The model under review builds one solid part; all positions refer to its coordinate system, in mm. Face numbers are marked on the shaded views. Round coordinates to 2 decimals unless told otherwise and drop trailing zeros. Loops run counter-clockwise (first coordinate to the right, second up) from the corner with the lowest first, then second, coordinate; pieces in that order, holes last. Notation, with made-up numbers: (-32.5, -18.75) -> (-6.5, -18.75) arc R14 ccw to (-6.5, -4.75) -> close; hole circle Ø7 at (3.5, 51). An arc over 180 degrees is marked (long way). Return JSON: item names as keys, results as strings. Group by question number.
```python
from build123d import *

# Parameters (mm, degrees)
F0_R     = 4.493782
F0_R_2   = 8.414158
F0_R_3   = 6.15385
F0_R_4   = 6.841255
F1_DEPTH = 6.35


with BuildPart() as f1:
    # F0 (on Front) → F1 (new body, symmetric)
    with BuildSketch(Plane.XZ):
        with BuildLine():
            Line((0, 9.352685), (0, 69.849999))
            ThreePointArc((0, 69.849999), (-26.730437, 64.532984), (-49.391408, 49.391408))
            Line((-49.391408, 49.391408), (-6.613347, 6.613347))
            ThreePointArc((-6.613347, 6.613347), (-3.579118, 8.640754), (0, 9.352685))
        make_face()
        with Locations((-9.287155, 20.851616)):
            Circle(F0_R, mode=Mode.SUBTRACT)
        with Locations((-19.314256, 38.508028)):
            Circle(F0_R_2, mode=Mode.SUBTRACT)
        with Locations((-36.098748, 50.714932)):
            Circle(F0_R_3, mode=Mode.SUBTRACT)
        with Locations((-12.992823, 59.434153)):
            Circle(F0_R_4, mode=Mode.SUBTRACT)
        with BuildLine():
            Line((7.121327, 6.062955), (49.917759, 48.859387))
            ThreePointArc((49.917759, 48.859387), (27.075766, 64.388859), (0, 69.849999))
            Line((0, 69.849999), (0, 9.352685))
            ThreePointArc((0, 9.352685), (3.922232, 8.490513), (7.121327, 6.062955))
        make_face()
        with Locations((9.287155, 20.851616)):
            Circle(F0_R, mode=Mode.SUBTRACT)
        with Locations((19.314256, 38.508028)):
            Circle(F0_R_2, mode=Mode.SUBTRACT)
        with Locations((36.098748, 50.714932)):
            Circle(F0_R_3, mode=Mode.SUBTRACT)
        with Locations((12.992823, 59.434153)):
            Circle(F0_R_4, mode=Mode.SUBTRACT)
        with BuildLine():
            Line((48.668913, 0), (69.849999, 0))
            ThreePointArc((69.849999, 0), (64.675257, 26.384341), (49.917759, 48.859387))
            Line((49.917759, 48.859387), (7.121327, 6.062955))
            ThreePointArc((7.121327, 6.062955), (8.777136, 3.230262), (9.352685, 0))
            Line((9.352685, 0), (33.899703, 0))
            ThreePointArc((33.899703, 0), (41.284308, 7.384605), (48.668913, 0))
        make_face()
        with Locations((21.909988, 8.228783)):
            Circle(F0_R, mode=Mode.SUBTRACT)
        with Locations((39.5664, 18.255884)):
            Circle(F0_R_2, mode=Mode.SUBTRACT)
        with Locations((60.492525, 11.934451)):
            Circle(F0_R_4, mode=Mode.SUBTRACT)
        with Locations((51.773304, 35.040376)):
            Circle(F0_R_3, mode=Mode.SUBTRACT)
        with BuildLine():
            ThreePointArc((57.120882, -40.202329), (66.591726, -21.084696), (69.849999, 0))
            Line((69.849999, 0), (48.668913, 0))
            ThreePointArc((48.668913, 0), (41.284308, -7.384605), (33.899703, 0))
            Line((33.899703, 0), (9.352685, 0))
            ThreePointArc((9.352685, 0), (8.640754, -3.579118), (6.613347, -6.613347))
            Line((6.613347, -6.613347), (49.391408, -49.391408))
            ThreePointArc((49.391408, -49.391408), (53.037147, -45.45419), (56.369892, -41.248728))
            ThreePointArc((56.369892, -41.248728), (46.021931, -34.968153), (57.927155, -37.15712))
            ThreePointArc((57.927155, -37.15712), (57.722172, -38.732189), (57.120882, -40.202329))
        make_face()
        with Locations((21.909988, -10.345527)):
            Circle(F0_R, mode=Mode.SUBTRACT)
        with Locations((39.5664, -20.372628)):
            Circle(F0_R_2, mode=Mode.SUBTRACT)
        with Locations((60.492525, -14.051196)):
            Circle(F0_R_4, mode=Mode.SUBTRACT)
        with BuildLine():
            ThreePointArc((41.248728, -56.369892), (45.45419, -53.037147), (49.391408, -49.391408))
            Line((49.391408, -49.391408), (6.613347, -6.613347))
            ThreePointArc((6.613347, -6.613347), (3.579118, -8.640754), (0, -9.352685))
            Line((0, -9.352685), (0, -69.849999))
            ThreePointArc((0, -69.849999), (21.084696, -66.591726), (40.202329, -57.120882))
            ThreePointArc((40.202329, -57.120882), (31.836894, -48.680561), (43.310971, -51.773304))
            ThreePointArc((43.310971, -51.773304), (42.771789, -54.292305), (41.248728, -56.369892))
        make_face()
        with Locations((14.051196, -60.492525)):
            Circle(F0_R_4, mode=Mode.SUBTRACT)
        with Locations((20.372628, -39.5664)):
            Circle(F0_R_2, mode=Mode.SUBTRACT)
        with Locations((10.345527, -21.909988)):
            Circle(F0_R, mode=Mode.SUBTRACT)
        with BuildLine():
            ThreePointArc((-48.859387, -49.917759), (-26.384341, -64.675257), (0, -69.849999))
            Line((0, -69.849999), (0, -9.352685))
            ThreePointArc((0, -9.352685), (-3.230262, -8.777136), (-6.062955, -7.121327))
            Line((-6.062955, -7.121327), (-48.859387, -49.917759))
        make_face()
        with Locations((-11.934451, -60.492525)):
            Circle(F0_R_4, mode=Mode.SUBTRACT)
        with Locations((-35.040376, -51.773304)):
            Circle(F0_R_3, mode=Mode.SUBTRACT)
        with Locations((-18.255884, -39.5664)):
            Circle(F0_R_2, mode=Mode.SUBTRACT)
        with Locations((-8.228783, -21.909988)):
            Circle(F0_R, mode=Mode.SUBTRACT)
        with BuildLine():
            ThreePointArc((-69.849999, 0), (-64.388859, -27.075766), (-48.859387, -49.917759))
            Line((-48.859387, -49.917759), (-6.062955, -7.121327))
            ThreePointArc((-6.062955, -7.121327), (-8.490513, -3.922232), (-9.352685, 0))
            Line((-9.352685, 0), (-33.899703, 0))
            ThreePointArc((-33.899703, 0), (-41.284308, -7.384605), (-48.668913, 0))
            Line((-48.668913, 0), (-69.849999, 0))
        make_face()
        with Locations((-50.714932, -36.098748)):
            Circle(F0_R_3, mode=Mode.SUBTRACT)
        with Locations((-38.508028, -19.314256)):
            Circle(F0_R_2, mode=Mode.SUBTRACT)
        with Locations((-59.434153, -12.992823)):
            Circle(F0_R_4, mode=Mode.SUBTRACT)
        with Locations((-20.851616, -9.287155)):
            Circle(F0_R, mode=Mode.SUBTRACT)
        with BuildLine():
            Line((-6.613347, 6.613347), (-49.391408, 49.391408))
            ThreePointArc((-49.391408, 49.391408), (-64.532984, 26.730437), (-69.849999, 0))
            Line((-69.849999, 0), (-48.668913, 0))
            ThreePointArc((-48.668913, 0), (-41.284308, 7.384605), (-33.899703, 0))
            Line((-33.899703, 0), (-9.352685, 0))
            ThreePointArc((-9.352685, 0), (-8.640754, 3.579118), (-6.613347, 6.613347))
        make_face()
        with Locations((-59.434153, 12.992823)):
            Circle(F0_R_4, mode=Mode.SUBTRACT)
        with Locations((-38.508028, 19.314256)):
            Circle(F0_R_2, mode=Mode.SUBTRACT)
        with Locations((-50.714932, 36.098748)):
            Circle(F0_R_3, mode=Mode.SUBTRACT)
        with Locations((-20.851616, 9.287155)):
            Circle(F0_R, mode=Mode.SUBTRACT)
    extrude(amount=F1_DEPTH, both=True)


solid = f1.part
```
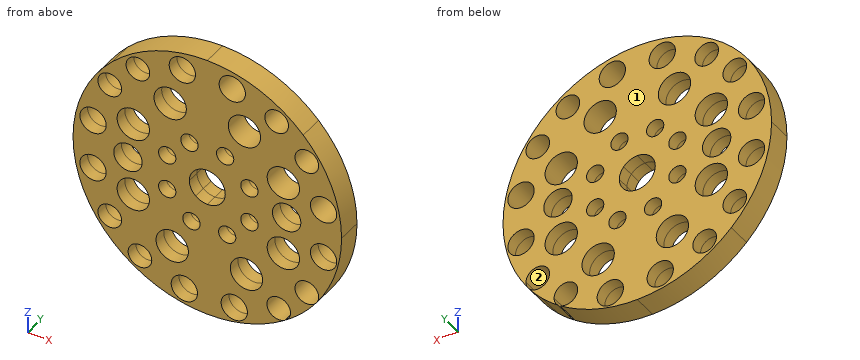
1. We need section A-A, the plane x = 23.5. Write out the cut boundary in (y, z).
2. We need section C-C, the plane y = 3. Give the number of separate pieces and of enclosed holes in the cut face, then the cut area to 3 significant figures.
3. Wall thickness on line 1 (X direction, y = -2, z = 25.5); line 2 (X direction, y = 1.75, z = -21); line 3 (X direction, y = 0.75, z = -49.5): over which ranges is each line inside the solid? List them lowest first.
4. For P1, Ø10, axis at x = -38.51, z = -19.31, coming from the -Y side; P2, Ø3, axis at x = -32.5, y = -1.5, coming from the +Z side; P3, Ø1.5, axis at x = -50.5, y = 4, coming from the +Z side, all flat-tipped, find the tip position at first contact; note any pin that passes through.
5. Draft analysis for pull direction Z (two halves, no side actions). For the marked faces 1 and 2, state which applies: pulls with the +Z half, pulls with the -Z half, needs draft (parallel to the pull), parting line crosses it, or undercut.
6. We need section B-B, the plane x = -23. Write out the cut boundary in (y, z), then the cut area to 3 significant figures.
Check sheet entries:
{
 "1": {"outline": "(-6.35, -65.78) -> (6.35, -65.78) -> (6.35, -47.38) -> (-6.35, -47.38) -> close; (-6.35, -31.76) -> (6.35, -31.76) -> (6.35, -14.55) -> (-6.35, -14.55) -> close; (-6.35, -6.14) -> (6.35, -6.14) -> (6.35, 4.03) -> (-6.35, 4.03) -> close; (-6.35, 12.43) -> (6.35, 12.43) -> (6.35, 31.21) -> (-6.35, 31.21) -> close; (-6.35, 45.81) -> (6.35, 45.81) -> (6.35, 65.78) -> (-6.35, 65.78) -> close"},
 "2": {"separate pieces": "1", "enclosed holes": "33", "area": "10,300 mm²"},
 "3": {"line 1": "x = -65.03 to -44.21, -32.8 to 35.29, 43.85 to 65.03", "line 2": "x = -66.62 to -46.75, -30.26 to -12.63, -3.83 to 5.94, 14.75 to 31.18, 47.96 to 66.62", "line 3": "x = -49.28 to -40.76, -29.32 to 31.44, 42.88 to 49.28"},
 "4": {"P1": "passes through", "P2": "stops at z = 62.59", "P3": "stops at z = 49.03"},
 "5": {"face 1": "needs draft", "face 2": "undercut"},
 "6": {"outline": "(-6.35, -65.95) -> (6.35, -65.95) -> (6.35, -46.52) -> (-6.35, -46.52) -> close; (-6.35, -32.62) -> (6.35, -32.62) -> (6.35, -13.23) -> (-6.35, -13.23) -> close; (-6.35, -5.34) -> (6.35, -5.34) -> (6.35, 5.34) -> (-6.35, 5.34) -> close; (-6.35, 13.23) -> (6.35, 13.23) -> (6.35, 30.94) -> (-6.35, 30.94) -> close; (-6.35, 46.07) -> (6.35, 46.07) -> (6.35, 65.95) -> (-6.35, 65.95) -> close", "area": "1,110 mm²"}
}
